Verification items for the finished model (mm, model axes). A direction names the side the tool comes from. Coordinates: 2 decimals unless noted, no trailing zeros. Write each loop counter-clockwise with the first axis right and the second up, starting at its lowest first coordinate (ties: lowest second). Pieces come first, ordered by that corner, then holes. Notation, with made-up numbers: M 5,32.25 L 27,32.25 A19 cw 27,66.25 Z; hole C 68,73.5 d4. An arc over 180 degrees is marked long. One line per item, written item: value.
```python
from build123d import *

# Parameters (mm, degrees)
BOSS_EXTRUDE1_DEPTH = 33
SKETCH2_R           = 1.25
BOSS_EXTRUDE2_DEPTH = 10
SKETCH3_R           = 1.25
CUT_EXTRUDE1_DEPTH  = 10


with BuildPart() as part:
    # Sketch1 → Boss-Extrude1 (new body)
    with BuildSketch(Plane(origin=(0, 0, 0), x_dir=(1, 0, 0), z_dir=(0, 1, 0))):
        Polygon((1.154700538, -2), (2.309401077, 0), (1.154700538, 2), (-1.154700538, 2), (-2.309401077, 0), (-1.154700538, -2), align=None)
    extrude(amount=BOSS_EXTRUDE1_DEPTH)

    # Sketch2 → Boss-Extrude2 (add)
    with BuildSketch(Plane(origin=(0, 0, 0), x_dir=(1, 0, 0), z_dir=(0, 1, 0))):
        with Locations(Location((0, 0, 0), (0, 0, 270))):
            Circle(SKETCH2_R)
    extrude(amount=-BOSS_EXTRUDE2_DEPTH)

    # Sketch3 → Cut-Extrude1 (cut)
    with BuildSketch(Plane(origin=(0, 33, 0), x_dir=(1, 0, 0), z_dir=(0, 1, 0))):
        with Locations(Location((0, 0, 0), (0, 0, 270))):
            Circle(SKETCH3_R)
    extrude(amount=-CUT_EXTRUDE1_DEPTH, mode=Mode.SUBTRACT)


solid = part.part
```
Item 1: Draft check along Z on faces 1 (the face through (0, 23, 0)), 2 (the face through (-1.22, -4.93, -0.27)), 3 (the face through (1, 0, -1)), 4 (the face through (0, 16, -2)). Enter one of: released by +Z, released by -Z, zero draft, split by the parting line, or undercut.
The answers:
face 1: undercut
face 2: split by the parting line
face 3: zero draft
face 4: released by -Z
Item 2: Cross-section at C-C, the plane z = -0.7. Enter the section's corners in (x, y).
The answers:
outline: M -1.91,0 L -1.04,0 L -1.04,-10 L 1.04,-10 L 1.04,0 L 1.91,0 L 1.91,33 L 1.04,33 L 1.04,23 L -1.04,23 L -1.04,33 L -1.91,33 Z
Item 3: Scan lines: line 1 (X direction, y = 30, z = 0); line 2 (Z direction, x = 0.5, y = 31); line 3 (Y direction, x = 1, z = 0.2). Record each from-to range of solid material in increasing order.
The answers:
line 1: x = -2.31 to -1.25, 1.25 to 2.31
line 2: z = -2 to -1.15, 1.15 to 2
line 3: y = -10 to 23
Item 4: Go/stop test with a flat-tipped pin: P1, Ø1, axis at y = -3, z = 1, coming from the -X side. Record where the tip stops, or that it passes through.
The answers:
P1: stops at x = -1.15
Item 5: Cross-section at A-A, the plane y = 26. Enter the section's corners in (x, z).
The answers:
outline: M -2.31,0 L -1.15,-2 L 1.15,-2 L 2.31,0 L 1.15,2 L -1.15,2 Z; hole C 0,0 d2.5
Item 6: Cross-section at B-B, the plane x = 0. Enter the section's corners in (y, z), and give its area (3 significant figures).
The answers:
outline: M -10,-1.25 L 0,-1.25 L 0,-2 L 33,-2 L 33,-1.25 L 23,-1.25 L 23,1.25 L 33,1.25 L 33,2 L 0,2 L 0,1.25 L -10,1.25 Z
area: 132 mm²
Item 7: Cross-section at D-D, the plane y = -4.5. Enter the section's corners in (x, z).
The answers:
outline: C 0,0 d2.5
Item 8: Access from +Z, -Z, +X, -X, +Y, -Y to the whole of each face (thin tool, end or side, straight path). Record for faces 5 (the face through (1.74, 16.27, -0.99)), 6 (the face through (-1.22, 28.07, -0.27)).
The answers:
face 5: -Z, +X, +Y, -Y
face 6: +Y
